from build123d import *

# Parameters (mm, degrees)
F2_DEPTH = 267.5


# Not quite as in the source:
# - ends of sketch curves that miss each other by under 0.0002 mm in the source are joined


with BuildPart() as f2:
    # F1 (on Front) → F2 (new body, symmetric)
    with BuildSketch(Plane.XZ):
        with BuildLine():
            Line((-8.250056, 12.999986), (-4.300056, 12.999986))
            ThreePointArc((-4.300056, 12.999986), (-4.0879239656, 13.0878539656), (-4.000056, 13.299986))
            Line((-4.000056, 13.299986), (-4.000056, 14.699986))
            ThreePointArc((-4.000056, 14.699986), (-4.0879239656, 14.9121180344), (-4.300056, 14.999986))
            Line((-4.300056, 14.999986), (-13.000056, 14.999986))
            ThreePointArc((-13.000056, 14.999986), (-14.4142695624, 14.4141995624), (-15.000056, 12.999986))
            Line((-15.000056, 12.999986), (-15.000056, 4.299986))
            ThreePointArc((-15.000056, 4.299986), (-14.9121880344, 4.0878539656), (-14.700056, 3.999986))
            Line((-14.700056, 3.999986), (-13.300056, 3.999986))
            ThreePointArc((-13.300056, 3.999986), (-13.0879239656, 4.0878539656), (-13.000056, 4.299986))
            Line((-13.000056, 4.299986), (-13.000056, 8.249986))
            Line((-13.000056, 8.249986), (-9.66427, 8.249986))
            Line((-9.66427, 8.249986), (-6.000056, 4.585772))
            Line((-6.000056, 4.585772), (-6.000056, 0.653576))
            ThreePointArc((-6.000056, 0.653576), (-5.9830189324, 0.5241665494), (-5.9330687764, 0.4035761291))
            Line((-5.9330687764, 0.4035761291), (-5.700056, -1.4e-05))
            Line((-5.700056, -1.4e-05), (-5.933069, -0.403604))
            ThreePointArc((-5.933069, -0.403604), (-6.000056, -0.653604), (-5.9330687764, -0.9036038709))
            Line((-5.9330687764, -0.9036038709), (-5.751033, -1.2189))
            Line((-5.751033, -1.2189), (-6.000056, -2.500014))
            Line((-6.000056, -2.500014), (-6.000056, -4.5858))
            Line((-6.000056, -4.5858), (-9.66427, -8.250014))
            Line((-9.66427, -8.250014), (-13.000056, -8.250014))
            Line((-13.000056, -8.250014), (-13.000056, -4.300014))
            ThreePointArc((-13.000056, -4.300014), (-13.0879239656, -4.0878819656), (-13.300056, -4.000014))
            Line((-13.300056, -4.000014), (-14.700056, -4.000014))
            ThreePointArc((-14.700056, -4.000014), (-14.9121880344, -4.0878819656), (-15.000056, -4.300014))
            Line((-15.000056, -4.300014), (-15.000056, -13.000014))
            ThreePointArc((-15.000056, -13.000014), (-14.4142695624, -14.4142275624), (-13.000056, -15.000014))
            Line((-13.000056, -15.000014), (12.999944, -15.000014))
            ThreePointArc((12.999944, -15.000014), (14.4141575624, -14.4142275624), (14.999944, -13.000014))
            Line((14.999944, -13.000014), (14.999944, 12.999986))
            ThreePointArc((14.999944, 12.999986), (14.4141575624, 14.4141995624), (12.999944, 14.999986))
            Line((12.999944, 14.999986), (4.299944, 14.999986))
            ThreePointArc((4.299944, 14.999986), (4.0878119656, 14.9121180344), (3.999944, 14.699986))
            Line((3.999944, 14.699986), (3.999944, 13.299986))
            ThreePointArc((3.999944, 13.299986), (4.0878119656, 13.0878539656), (4.299944, 12.999986))
            Line((4.299944, 12.999986), (8.249944, 12.999986))
            Line((8.249944, 12.999986), (8.249944, 9.6642))
            Line((8.249944, 9.6642), (4.58573, 5.999986))
            Line((4.58573, 5.999986), (0.653534, 5.999986))
            ThreePointArc((0.653534, 5.999986), (0.5241245494, 5.9829489324), (0.4035341291, 5.9329987764))
            Line((0.4035341291, 5.9329987764), (-5.6e-05, 5.699986))
            Line((-5.6e-05, 5.699986), (-0.403646, 5.932999))
            ThreePointArc((-0.403646, 5.932999), (-0.653646, 5.999986), (-0.9036458709, 5.9329987764))
            Line((-0.9036458709, 5.9329987764), (-1.218942, 5.750963))
            Line((-1.218942, 5.750963), (-2.500056, 5.999986))
            Line((-2.500056, 5.999986), (-4.585842, 5.999986))
            Line((-4.585842, 5.999986), (-8.250056, 9.6642))
            Line((-8.250056, 9.6642), (-8.250056, 12.999986))
        make_face()
        with BuildLine():
            ThreePointArc((-8.189375, -13.000014), (-8.339375082, -12.9598215738), (-8.4491827159, -12.8500138359))
            ThreePointArc((-8.4491827159, -12.8500138359), (-9.2743948384, -12.3508472042), (-10.1375690315, -12.7810479782))
            ThreePointArc((-10.1375690315, -12.7810479782), (-13.2041723505, -12.8608903949), (-12.3498940253, -9.9145979306))
            Line((-12.3498940253, -9.9145979306), (-11.07346, -9.450014))
            Line((-11.07346, -9.450014), (-8.450056, -9.450014))
            ThreePointArc((-8.450056, -9.450014), (-8.0673725676, -9.3738935325), (-7.7429492188, -9.1571207812))
            Line((-7.7429492188, -9.1571207812), (-4.878736, -6.292907))
            ThreePointArc((-4.878736, -6.292907), (-4.5543124324, -6.0761344675), (-4.171629, -6.000014))
            Line((-4.171629, -6.000014), (4.171517, -6.000014))
            ThreePointArc((4.171517, -6.000014), (4.5542004324, -6.0761344675), (4.8786237812, -6.2929072188))
            Line((4.8786237812, -6.2929072188), (7.957051, -9.371334))
            ThreePointArc((7.957051, -9.371334), (8.1738235325, -9.6957575676), (8.249944, -10.078441))
            Line((8.249944, -10.078441), (8.249944, -12.000014))
            ThreePointArc((8.249944, -12.000014), (7.9570507812, -12.7071207812), (7.249944, -13.000014))
            Line((7.249944, -13.000014), (-8.189375, -13.000014))
        make_face(mode=Mode.SUBTRACT)
        with BuildLine():
            ThreePointArc((9.5477956661, -11.3422641215), (9.8734155063, -9.8734855063), (11.3421941215, -9.5478656661))
            Line((11.3421941215, -9.5478656661), (12.349782, -9.914598))
            ThreePointArc((12.349782, -9.914598), (13.0434468843, -13.0435168843), (9.9145279306, -12.3498520253))
            Line((9.9145279306, -12.3498520253), (9.5477956661, -11.3422641215))
        make_face(mode=Mode.SUBTRACT)
        with BuildLine():
            ThreePointArc((-9.5479076661, 11.3422361215), (-9.8735275063, 9.8734575063), (-11.3423061215, 9.5478376661))
            Line((-11.3423061215, 9.5478376661), (-12.349894, 9.91457))
            ThreePointArc((-12.349894, 9.91457), (-13.0435588843, 13.0434888843), (-9.9146399306, 12.3498240253))
            Line((-9.9146399306, 12.3498240253), (-9.5479076661, 11.3422361215))
        make_face(mode=Mode.SUBTRACT)
        with BuildLine():
            ThreePointArc((3.2531309855, 0.9883049956), (3.399944, -1.4e-05), (3.2531309855, -0.9883329956))
            ThreePointArc((3.2531309855, -0.9883329956), (3.2974111593, -1.3177976431), (3.5754529349, -1.5000144258))
            ThreePointArc((3.5754529349, -1.5000144258), (3.8792555231, -1.6685151025), (3.999944, -1.99428))
            Line((3.999944, -1.99428), (3.999944, -3.500014))
            ThreePointArc((3.999944, -3.500014), (3.8534973906, -3.8535673906), (3.499944, -4.000014))
            Line((3.499944, -4.000014), (1.99421, -4.000014))
            ThreePointArc((1.99421, -4.000014), (1.6684451025, -3.8793255231), (1.4999444822, -3.5755229263))
            ThreePointArc((1.4999444822, -3.5755229263), (1.3177276431, -3.2974811593), (0.9882590481, -3.2532021585))
            ThreePointArc((0.9882590481, -3.2532021585), (-5.6e-05, -3.400014), (-0.9883749956, -3.2532009855))
            ThreePointArc((-0.9883749956, -3.2532009855), (-1.3178396431, -3.2974811593), (-1.5000564258, -3.5755229349))
            ThreePointArc((-1.5000564258, -3.5755229349), (-1.6685571025, -3.8793255231), (-1.994322, -4.000014))
            Line((-1.994322, -4.000014), (-3.500056, -4.000014))
            ThreePointArc((-3.500056, -4.000014), (-3.8536093906, -3.8535673906), (-4.000056, -3.500014))
            Line((-4.000056, -3.500014), (-4.000056, -1.99428))
            ThreePointArc((-4.000056, -1.99428), (-3.8793675231, -1.6685151025), (-3.5755649263, -1.5000144822))
            ThreePointArc((-3.5755649263, -1.5000144822), (-3.2975231593, -1.3177976431), (-3.2532441585, -0.9883290481))
            ThreePointArc((-3.2532441585, -0.9883290481), (-3.400056, -1.4e-05), (-3.2532429855, 0.9883049956))
            ThreePointArc((-3.2532429855, 0.9883049956), (-3.2975231593, 1.3177696431), (-3.5755649349, 1.4999864258))
            ThreePointArc((-3.5755649349, 1.4999864258), (-3.8793675231, 1.6684871025), (-4.000056, 1.994252))
            Line((-4.000056, 1.994252), (-4.000056, 3.499986))
            ThreePointArc((-4.000056, 3.499986), (-3.8536093906, 3.8535393906), (-3.500056, 3.999986))
            Line((-3.500056, 3.999986), (-1.994322, 3.999986))
            ThreePointArc((-1.994322, 3.999986), (-1.6685571025, 3.8792975231), (-1.5000564822, 3.5754949263))
            ThreePointArc((-1.5000564822, 3.5754949263), (-1.3178396431, 3.2974531593), (-0.9883710481, 3.2531741585))
            ThreePointArc((-0.9883710481, 3.2531741585), (-5.6e-05, 3.399986), (0.9882629956, 3.2531729855))
            ThreePointArc((0.9882629956, 3.2531729855), (1.3177276431, 3.2974531593), (1.4999444258, 3.5754949349))
            ThreePointArc((1.4999444258, 3.5754949349), (1.6684451025, 3.8792975231), (1.99421, 3.999986))
            Line((1.99421, 3.999986), (3.499944, 3.999986))
            ThreePointArc((3.499944, 3.999986), (3.8534973906, 3.8535393906), (3.999944, 3.499986))
            Line((3.999944, 3.499986), (3.999944, 1.994252))
            ThreePointArc((3.999944, 1.994252), (3.8792555231, 1.6684871025), (3.5754529263, 1.4999864822))
            ThreePointArc((3.5754529263, 1.4999864822), (3.2974111593, 1.3177696431), (3.2531309855, 0.9883049956))
        make_face(mode=Mode.SUBTRACT)
        with BuildLine():
            ThreePointArc((6.2928372188, -4.8786937812), (6.0760644675, -4.5542704324), (5.999944, -4.171587))
            Line((5.999944, -4.171587), (5.999944, 4.171559))
            ThreePointArc((5.999944, 4.171559), (6.0760644675, 4.5542424324), (6.2928372188, 4.8786657812))
            Line((6.2928372188, 4.8786657812), (9.157051, 7.742879))
            ThreePointArc((9.157051, 7.742879), (9.3738235325, 8.0673025676), (9.449944, 8.449986))
            Line((9.449944, 8.449986), (9.449944, 11.07339))
            Line((9.449944, 11.07339), (9.914528, 12.349824))
            ThreePointArc((9.914528, 12.349824), (12.8608203949, 13.2041023505), (12.7809779799, 10.1374990291))
            ThreePointArc((12.7809779799, 10.1374990291), (12.3507772042, 9.2743248384), (12.8499438252, 8.4491126972))
            ThreePointArc((12.8499438252, 8.4491126972), (12.9597515738, 8.339305082), (12.999944, 8.189305))
            Line((12.999944, 8.189305), (12.999944, -7.250014))
            ThreePointArc((12.999944, -7.250014), (12.7070507812, -7.9571207812), (11.999944, -8.250014))
            Line((11.999944, -8.250014), (10.078371, -8.250014))
            ThreePointArc((10.078371, -8.250014), (9.6956875676, -8.1738935325), (9.3712642188, -7.9571207812))
            Line((9.3712642188, -7.9571207812), (6.2928372188, -4.8786937812))
        make_face(mode=Mode.SUBTRACT)
    extrude(amount=F2_DEPTH, both=True)


solid = f2.part
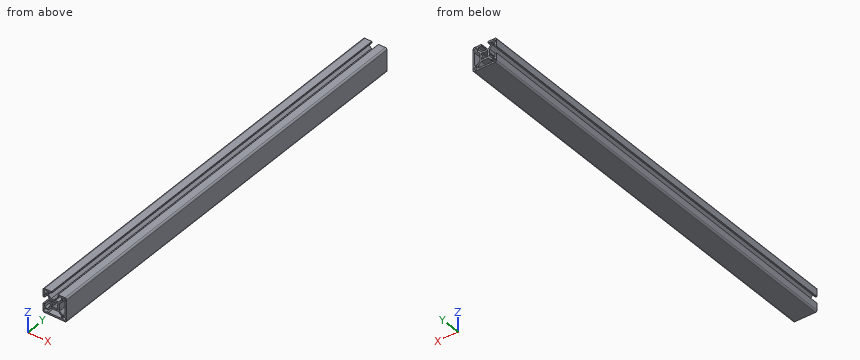
Geometry: final body of the model. Coordinates: model frame, mm. Give positions to 0.01 mm unless a question says otherwise; leave off trailing zeros. Answer as CSV lines item,"result". Start each with the question number.
1. Pin query (flat end, axial travel): P1, Ø0.7, axis at x = -14, y = -94, coming from the +Z side; P2, Ø1.7, axis at y = -5.5, z = -3, coming from the -X side; P3, Ø1.7, axis at x = 3, y = -15.5, coming from the +Z side. Return the tip coordinate at first contact, or that it passes through.
2. Section A-A, the plane y = -221. Give the number of separate pieces and of enclosed holes in the cut face, plus the area to 3 significant figures.
3. Ray query, L1, parallel to X at y = 198.5, z = 9.25; L2, parallel to X at y = -54, z = 2.5; L3, parallel to Z at x = 10.25, y = -91.5. Return the intervals inside material, ascending.
Answers:
1,P1,"stops at z = 14.89"
1,P2,"stops at x = -6"
1,P3,"stops at z = 6"
2,separate pieces,"1"
2,enclosed holes,"5"
2,area,"339 mm2"
3,L1,"x = -15 to -7.84, 7.84 to 9.45, 12.35 to 15"
3,L2,"x = -6 to -4, 4 to 6, 13 to 15"
3,L3,"z = -15 to -12.93, -9.6 to -8.25, 12.93 to 15"
